Autodesk Inventor part; units mm, degrees
ref_plane "YZ Plane" through (0, 0, 0) normal (1, 0, 0) x (0, 1, 0)
ref_plane "XZ Plane" through (0, 0, 0) normal (0, 1, 0) x (-1, 0, 0)
ref_plane "XY Plane" through (0, 0, 0) normal (0, 0, 1) x (1, 0, 0)
sketch "Esquisse1" plane through (0, 0, 0) normal (0, 0, 1) x (1, 0, 0)
  line L0 (-192.7, -147.2) -> (192.7, -147.2)
  line L1 (192.7, -147.2) -> (192.7, 147.2)
  line L2 (192.7, 147.2) -> (-192.7, 147.2)
  line L3 (-192.7, 147.2) -> (-192.7, -147.2)
  line L4 (-192.7, -147.2) -> (192.7, 147.2) construction
  line L5 (192.7, -147.2) -> (-192.7, 147.2) construction
  point P0 (0, 0)
  dimension "Largueur_plaque_inf" = 385.4
  dimension "Profondeur_plaque_inf" = 294.4
extrude "Embase" add sketch "Esquisse1" along normal mid plane 5
sketch "Esquisse2" plane through (0, 0, 2.5) normal (0, 0, 1) x (1, 0, 0)
  point P0 (0, 0)
  point P1 (-53, -127)
  dimension "d4" = 53
  dimension "d5" = 127
hole "Perçage" at (-53, -127, 2.5) direction (0, 0, -1) diameter 7.5 end through all
pattern_linear "Réseau rectangulaire largueur" count 7 spacing 18 along (1, 0, 0) of "Perçage"
pattern_linear "Réseau rectangulaire profondeur" count 10 spacing 19 along (0, 1, 0) of "Perçage", "Réseau rectangulaire largueur"
sketch "Esquisse3" plane through (0, 0, 2.5) normal (0, 0, 1) x (1, 0, 0)
  circle A0 centre (-192.7, 147.2) radius 25
  line L0 (192.7, 147.2) -> (-192.7, 147.2) construction
  line L1 (-192.7, 147.2) -> (-192.7, -147.2) construction
  point P0 (0, 0)
  dimension "d19" = 50
extrude "Passage cable" cut sketch "Esquisse3" against normal through all
fillet "Congé1" radius 10 2 edges at (-192.7, 122.2, 0) (-167.7, 147.2, 0)
properties part number "Plaque inferieur" material "Plastique PMMA"
The model under review builds one solid part; all positions refer to its coordinate system, in mm. Coordinates: 2 decimals unless noted, no trailing zeros.
1) To check wall thickness, follow probe 1 along Y at (x, z) = (-175.5, -1.75); probe 2 along X at (y, z) = (135, 1.05); probe 3 along Y at (x, z) = (-163, 2). State the ranges of each line that lie inside material, in increasing order.
2) We need section A-A on z = -0.4. Count the separate pieces of the cut face and the enclosed holes in it, then the cut area to 3 significant figures.
3) The part is to be moulded in two halves that separate along X. For faces 1 (the face through (-49.673, -109.73, -0.035)), 2 (the face through (-3, 2, -2.5)), say which applies: pulls with the +X half, pulls with the -X half, needs draft (parallel to the pull), parting line crosses it, or undercut.
4) Clearance check with flat-ended pins moving along their axes: pin 1 Ø6 at (x, y) = (-53, 44) entering from +Z; pin 2 Ø8.5 at (x, y) = (-53, -70) entering from +Z. State where each tip first meets the part, or that it passes through.
Answer list:
1. probe 1: y = -147.2 to 129.06
1. probe 2: x = -170.88 to 192.7
1. probe 3: y = -147.2 to 146.43
2. separate pieces: 1
2. enclosed holes: 70
2. area: 110,000 mm2
3. face 1: undercut
3. face 2: needs draft
4. pin 1: passes through
4. pin 2: stops at z = 2.5
